Design review of the part built by this model. Coordinates are the model's own, in mm. Coordinates: 2 decimals unless noted, no trailing zeros. Loops run counter-clockwise (first coordinate to the right, second up) from the corner with the lowest first, then second, coordinate; pieces in that order, holes last. Notation, with made-up numbers: M 10.25,85.25 L 59.25,85.25 A22 cw 59.25,108.25 Z; hole C 11,32 d6. An arc over 180 degrees is marked long. Put each result on its own line as item: value. Start each with the question number.
(1) For probe 1 along X at (y, z) = (123.5, 1.15); probe 2 along Y at (x, z) = (91, 1.4), list the stretches that pass through material, from the lowest coordinate up. Write a range as [from, to].
(2) Clearance check with flat-ended pins moving along their axes: pin 1 (1.5 mm diameter, centred on x = 88.5, z = 1, fed in from +Y); pin 2 (0.9 mm diameter, centred on y = 99.5, z = 1.5, fed in from +X); pin 3 (1 mm diameter, centred on y = 104.5, z = 2.5, fed in from -X); pin 4 (6 mm diameter, centred on x = 79.5, y = 120, fed in from -Z). State where each tip first meets the part, or that it passes through.
(3) Take a section at A-A, the plane z = 2.2. Give the boundary of the cut face in (x, y).
(4) Take a section at C-C, the plane x = 60.5. Give the boundary of the cut face in (y, z), then the cut area to 3 significant figures.
(5) Take a section at B-B, the plane y = 100.5. Give the boundary of the cut face in (x, z), then the cut area to 3 significant figures.
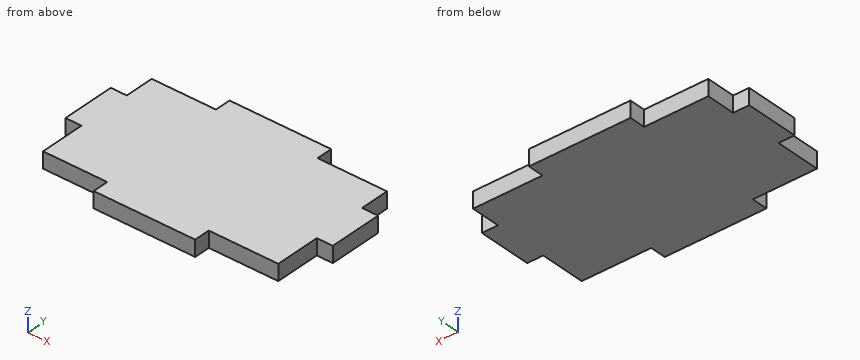
Autodesk Fusion 360 part; units mm, degrees
sketch "Sketch1" plane through (0, 0, 0) normal (0, 0, 1) x (1, 0, 0)
  line L0 (50, 125) -> (62, 125)
  line L1 (62, 125) -> (62, 128)
  line L2 (62, 128) -> (81, 128)
  line L3 (81, 128) -> (81, 125)
  line L4 (81, 125) -> (94, 125)
  line L5 (94, 125) -> (94, 119.5)
  line L6 (94, 119.5) -> (97, 119.5)
  line L7 (97, 119.5) -> (97, 109.5)
  line L8 (97, 109.5) -> (94, 109.5)
  line L9 (94, 109.5) -> (94, 101)
  line L10 (94, 101) -> (81, 101)
  line L11 (81, 101) -> (81, 98)
  line L12 (81, 98) -> (62, 98)
  line L13 (62, 98) -> (62, 101)
  line L14 (62, 101) -> (50, 101)
  line L15 (50, 101) -> (50, 109.5)
  line L16 (50, 109.5) -> (47, 109.5)
  line L17 (47, 109.5) -> (47, 119.5)
  line L18 (47, 119.5) -> (50, 119.5)
  line L19 (50, 119.5) -> (50, 125)
  dimension "d1" = 12
  dimension "d2" = 3
  dimension "d3" = 19
  dimension "d4" = 3
  dimension "d5" = 13
  dimension "d6" = 5.5
  dimension "d7" = 3
  dimension "d8" = 10
  dimension "d9" = 3
  dimension "d10" = 8.5
  dimension "d11" = 13
  dimension "d12" = 3
  dimension "d13" = 19
  dimension "d14" = 3
  dimension "d15" = 12
  dimension "d16" = 8.5
  dimension "d17" = 3
  dimension "d18" = 10
  dimension "d19" = 3
extrude "Extrude1" add sketch "Sketch1" along normal blind 3
Computed values:
1. probe 1: x = [50, 94]
1. probe 2: y = [101, 125]
2. pin 1: stops at y = 125
2. pin 2: stops at x = 81
2. pin 3: stops at x = 50
2. pin 4: stops at z = 0
3. outline: M 47,109.5 L 50,109.5 L 50,101 L 62,101 L 62,98 L 81,98 L 81,101 L 94,101 L 94,109.5 L 97,109.5 L 97,119.5 L 94,119.5 L 94,125 L 81,125 L 81,128 L 62,128 L 62,125 L 50,125 L 50,119.5 L 47,119.5 Z
4. outline: M 101,0 L 125,0 L 125,3 L 101,3 Z
4. area: 72.0 mm^2
5. outline: M 62,0 L 81,0 L 81,3 L 62,3 Z
5. area: 57.0 mm^2
